Verification items for this drawing (mm, ordinates from the low corner). A direction names the side the tool comes from. Give positions to 0.01 mm unless a question says otherwise; leave off trailing zeros. Order: outer loops, then holes, each group sorted by start corner. A loop starts at its lowest first (then second) coordinate and runs counter-clockwise, first axis right, second up. Notation, with made-up numbers: (47.5, -25) -> (77.5, -25) arc R32 cw to (77.5, 11) -> close; hole circle Ø6 at (5.5, 32.5). An arc over 180 degrees is marked (long way). One line per question, with ' | ' between items.
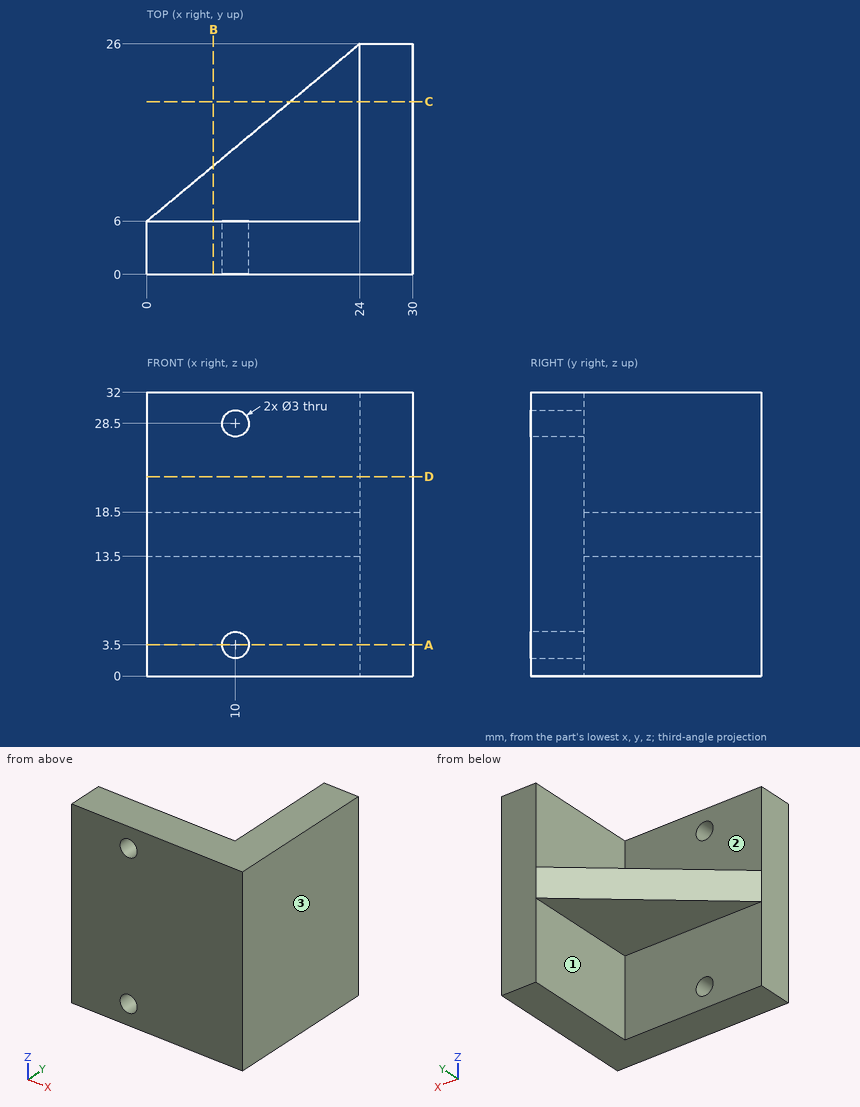
Q1. Access from +Z, -Z, +X, -X, +Y, -Y to the whole of each face (thin tool, end or side, straight path). Record for the marked faces 1, 2 and 3.
Result sheet:
face 1: -Z, -X, +Y | face 2: +Z, -X, +Y | face 3: +Z, -Z, +X, +Y, -Y
Q2. Thickness scan on line 1 (X direction, y = 3.5, z = 28.5); line 2 (X direction, y = 21.5, z = 30); line 3 (Y direction, x = 14, z = 23.5). Record the ranges inside material, lowest first.
Result sheet:
line 1: x = 0 to 8.5, 11.5 to 30 | line 2: x = 24 to 30 | line 3: y = 0 to 6
Q3. Section check B-B (x = 7.5). Enter the section's corners in (y, z), and give its area (3 significant figures).
Result sheet:
outline: (0, 0) -> (6, 0) -> (6, 13.5) -> (12.25, 13.5) -> (12.25, 18.5) -> (6, 18.5) -> (6, 32) -> (0, 32) -> close | area: 223 mm2
Q4. Section check C-C (y = 19.5). Enter the section's corners in (x, z).
Result sheet:
outline: (16.2, 13.5) -> (24, 13.5) -> (24, 0) -> (30, 0) -> (30, 32) -> (24, 32) -> (24, 18.5) -> (16.2, 18.5) -> close
Q5. Depth check by flat-ended pin: pin 1 Ø5 at (x, z) = (10, 28.5) entering from -Y; pin 2 Ø1 at (x, z) = (23, 12.5) entering from +Y; pin 3 Ø1.8 at (x, z) = (10, 3.5) entering from +Y; pin 4 Ø4 at (y, z) = (13.5, 24.5) entering from -X. Enter the tip coordinate at first touch or a pass-through.
Result sheet:
pin 1: stops at y = 0 | pin 2: stops at y = 6 | pin 3: passes through | pin 4: stops at x = 24
Q6. Section check D-D (z = 22.5). Enter the section's corners in (x, y).
Result sheet:
outline: (0, 0) -> (30, 0) -> (30, 26) -> (24, 26) -> (24, 6) -> (0, 6) -> close
Q7. Section check A-A (z = 3.5). Enter the section's corners in (x, y), and give its area (3 significant figures).
Result sheet:
outline: (0, 0) -> (8.5, 0) -> (8.5, 6) -> (0, 6) -> close; (11.5, 0) -> (30, 0) -> (30, 26) -> (24, 26) -> (24, 6) -> (11.5, 6) -> close | area: 282 mm2
